For this review, take the finished solid that the model builds, in its own axes (mm). Face numbers are marked on the shaded views. A direction names the side the tool comes from. Coordinates: 2 decimals unless noted, no trailing zeros. Write each loop counter-clockwise with the first axis right and the second up, starting at its lowest first coordinate (ties: lowest second). Pieces come first, ordered by that corner, then holes. Notation, with made-up numbers: (41.25, -32) - (65.25, -32) arc R23 cw to (65.25, -10) - close; hole circle Ø6 at (33.25, -38). An arc over 180 degrees is marked (long way). Use one line per item in the form item = value. Start each with the question number.
1) Mouldability with a two-part tool opening along X and no side actions: class the marked faces 4, 5 and 6 as pulls with the +X half, pulls with the -X half, needs draft (parallel to the pull), parting line crosses it, or undercut.
2) We need section B-B (z = 643). Give the boundary of the cut face in (x, y), plus the area to 3 significant figures.
3) Tool access review of the marked faces 1, 2 and 3: name each direction out of +Z, -Z, +X, -X, +Y, -Y from which nothing blocks a thin tool from reaching the whole face with its end or side.
4) Insertion check: P1, Ø4, axis at x = 246, z = 211.5, coming from the +Y side; P2, Ø8, axis at y = 168, z = 681, coming from the -X side; P3, Ø1.5, axis at x = 22, z = 289.5, coming from the +Y side. Each pin has a flat end and moves straight along its axis. Give the tip position at first contact, or say it passes through.
5) For L1, parallel to Y at x = 172.5, z = 539; L2, parallel to X at y = 90.5, z = 198; L3, parallel to X at y = 125.5, z = 416, list the stretches that pass through material, from the lowest coordinate up. Write a range as from..to.
6) We need section A-A (y = 162). Give the boundary of the cut face in (x, z), plus the area to 3 significant figures.
7) We need section C-C (x = 139). Give the boundary of the cut face in (y, z), plus the area to 3 significant figures.
```python
from build123d import *

# Parameters (mm, degrees)
BOSS_EXTRUDE1_DEPTH = 838.2
SKETCH4_W           = 57.15
SKETCH4_H           = 38.1
CUT_EXTRUDE3_DEPTH  = 2.54
SKETCH5_W           = 7.112
SKETCH5_H           = 69.85
CUT_EXTRUDE4_DEPTH  = 2.6002


with BuildPart() as part:
    # Sketch1 → Boss-Extrude1 (new body)
    with BuildSketch(Plane.XY):
        Polygon((-0.223728527, 63.622161409), (51.646062311, 189.021961409), (204.046062311, 189.021961409), (255.915853149, 63.622161409), (318.346062311, 63.622161409), (318.346062311, 62.021961409), (254.846062311, 62.021961409), (202.976271473, 187.421761409), (52.715853149, 187.421761409), (0.846062311, 62.021961409), (-62.653937689, 62.021961409), (-62.653937689, 63.622161409), align=None)
    extrude(amount=BOSS_EXTRUDE1_DEPTH)

    # Sketch4 → Cut-Extrude3 (cut)
    with BuildSketch(Plane(origin=(0, 63.622161409, 0), x_dir=(1, 0, 0), z_dir=(0, 1, 0))):
        with Locations((289.771062311, -382.905)):
            Rectangle(SKETCH4_W, SKETCH4_H)
        with Locations((289.771062311, -455.295)):
            Rectangle(SKETCH4_W, SKETCH4_H)
    extrude(amount=-CUT_EXTRUDE3_DEPTH, mode=Mode.SUBTRACT)

    # Sketch5 → Cut-Extrude4 (cut, through all)
    with BuildSketch(Plane(origin=(0, 63.622161409, 0), x_dir=(1, 0, 0), z_dir=(0, 1, 0))):
        with Locations((-27.093937689, -34.925)):
            Rectangle(SKETCH5_W, SKETCH5_H)
        with Locations((-39.793937689, -803.275)):
            Rectangle(SKETCH5_W, SKETCH5_H)
        with Locations((277.706062311, -34.925)):
            Rectangle(SKETCH5_W, SKETCH5_H)
        with Locations((303.106062311, -803.275)):
            Rectangle(SKETCH5_W, SKETCH5_H)
    extrude(amount=-CUT_EXTRUDE4_DEPTH, mode=Mode.SUBTRACT)


solid = part.part
```
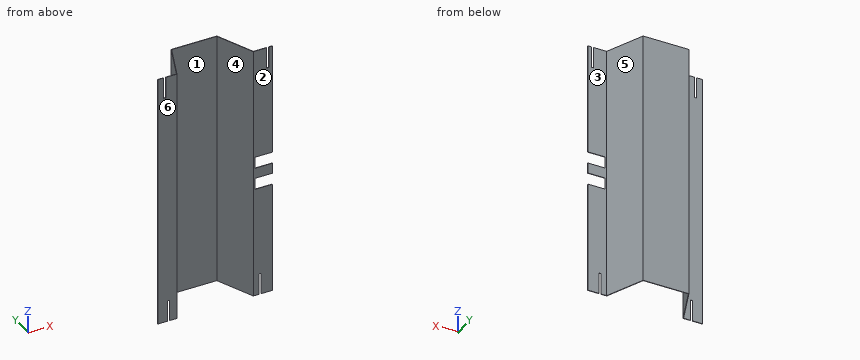
Determined:
q1.face_4 = undercut
q1.face_5 = pulls with the +X half
q1.face_6 = needs draft
q2.outline = (-62.65, 62.02) - (0.85, 62.02) - (52.72, 187.42) - (202.98, 187.42) - (254.85, 62.02) - (318.35, 62.02) - (318.35, 63.62) - (255.92, 63.62) - (204.05, 189.02) - (51.65, 189.02) - (-0.22, 63.62) - (-62.65, 63.62) - close
q2.area = 878 mm²
q3.face_1 = +Z, -Z, -Y
q3.face_2 = +Z, -Z, +X, -X, -Y
q3.face_3 = +Z, -Z, +X, +Y
q4.P1 = 92.43
q4.P2 = 41.3
q4.P3 = 119.16
q5.L1 = 187.42..189.02
q5.L2 = 10.89..12.63, 243.07..244.8
q5.L3 = 25.37..27.1, 228.59..230.32
q6.outline = (40.47, 0) - (42.2, 0) - (42.2, 838.2) - (40.47, 838.2) - close; (213.49, 0) - (215.22, 0) - (215.22, 838.2) - (213.49, 838.2) - close
q6.area = 2,900 mm²
q7.outline = (187.42, 0) - (189.02, 0) - (189.02, 838.2) - (187.42, 838.2) - close
q7.area = 1,340 mm²
